Drawing for the job (mm, zero at the part's lowest x, y, z). A direction names the side the tool comes from. Coordinates: 2 decimals unless noted, no trailing zeros. Write each loop counter-clockwise with the first axis right and the second up, starting at its lowest first coordinate (ties: lowest second). Pieces come first, ordered by that corner, then holes. Notation, with made-up numbers: (-6, 0.5) - (23, 0.5) arc R23 cw to (23, 30.5) - close; hole circle Ø2 at (73.25, -36). An arc over 180 degrees is marked (long way). Write each question's results on one line, items separated by ' | '.
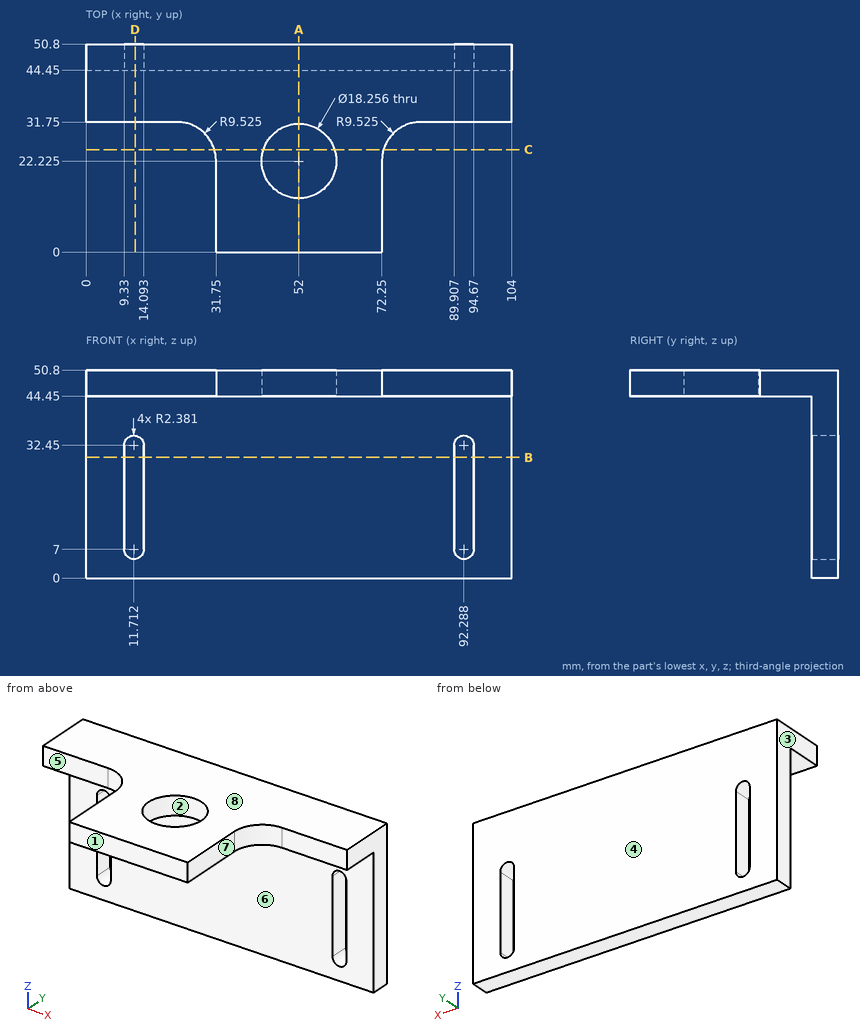
(1) Saw through at B-B on z = 29.5. Write the cut outline in (x, y).
Return value:
outline: (0, 44.45) - (9.33, 44.45) - (9.33, 50.8) - (0, 50.8) - close; (14.09, 44.45) - (89.91, 44.45) - (89.91, 50.8) - (14.09, 50.8) - close; (94.67, 44.45) - (104, 44.45) - (104, 50.8) - (94.67, 50.8) - close
(2) Two-plate mould, pull along Y, no slides. Class the marked faces 1, 2 and 3: released by +Y, released by -Y, zero draft, split by the parting line, or undercut.
Return value:
face 1: released by -Y | face 2: undercut | face 3: zero draft
(3) Wall check: line 1 (Y direction, x = 52, z = 48); line 2 (Y direction, x = 61, z = 35). Give the ranges that are in metal, low to high. Write a range as from..to.
Return value:
line 1: y = 0..13.1, 31.35..50.8 | line 2: y = 44.45..50.8
(4) Flat gauge pins, fed straight in: P1, Ø10, axis at x = 52.5, z = 7.5, coming from the -Y side; P2, Ø3, axis at x = 92, z = 46.5, coming from the -Y side; P3, Ø5, axis at y = 6.5, z = 47, coming from the -X side. Where does each tip first touch, or does it go through?
Return value:
P1: stops at y = 44.45 | P2: stops at y = 31.75 | P3: stops at x = 31.75
(5) Saw through at D-D on x = 12. Write the cut outline in (y, z), then the cut area to 3 significant figures.
Return value:
outline: (31.75, 44.45) - (44.45, 44.45) - (44.45, 34.81) - (50.8, 34.81) - (50.8, 50.8) - (31.75, 50.8) - close; (44.45, 0) - (50.8, 0) - (50.8, 4.64) - (44.45, 4.64) - close | area: 212 mm^2
(6) Saw through at C-C on y = 25. Write the cut outline in (x, z), then the cut area to 3 significant figures.
Return value:
outline: (31.34, 44.45) - (43.3, 44.45) - (43.3, 50.8) - (31.34, 50.8) - close; (60.7, 44.45) - (72.66, 44.45) - (72.66, 50.8) - (60.7, 50.8) - close | area: 152 mm^2
(7) Saw through at A-A on x = 52. Write the cut outline in (y, z), then the cut area to 3 significant figures.
Return value:
outline: (0, 44.45) - (13.1, 44.45) - (13.1, 50.8) - (0, 50.8) - close; (31.35, 44.45) - (44.45, 44.45) - (44.45, 0) - (50.8, 0) - (50.8, 50.8) - (31.35, 50.8) - close | area: 489 mm^2
(8) 3-axis set-ups, long thin cutter, end or side, ignore diameter. For the marked faces 4, 5, 6, 7 and 8: which of +Z, -Z, +X, -X, +Y, -Y reach the whole face in a straight line?
Return value:
face 4: +Z, -Z, +X, -X, +Y | face 5: +Z, -Z, -X, -Y | face 6: -Z, +X, -X, -Y | face 7: +Z, -Z, +X, -Y | face 8: +Z, +X, -X, +Y, -Y
